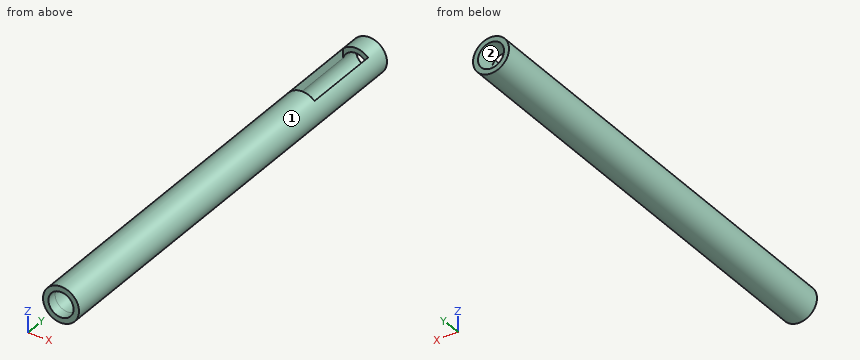
from build123d import *

# Parameters (mm, degrees)
SKETCH1_R           = 18
SKETCH1_R_2         = 13
BOSS_EXTRUDE1_DEPTH = 225
SKETCH8_R           = 18
BOSS_EXTRUDE3_DEPTH = 10
SKETCH9_R           = 12.55
CUT_EXTRUDE2_DEPTH  = 899.5
SKETCH23_W          = 25
SKETCH23_H          = 80
CUT_EXTRUDE16_DEPTH = 30


with BuildPart() as part:
    # Sketch1 → Boss-Extrude1 (new, symmetric)
    with BuildSketch(Plane(origin=(0, 0, 0), x_dir=(1, 0, 0), z_dir=(0, 1, 0))):
        with Locations(Location((0, 0, 0), (0, 0, 270))):
            Circle(SKETCH1_R)
        with Locations(Location((0, 0, 0), (0, 0, 270))):
            Circle(SKETCH1_R_2, mode=Mode.SUBTRACT)
    extrude(amount=BOSS_EXTRUDE1_DEPTH, both=True)

    # Sketch8 → Boss-Extrude3 (add)
    with BuildSketch(Plane.XZ.offset(225)):
        with Locations(Location((0, 0, 0), (0, 0, 270))):
            Circle(SKETCH8_R)
    extrude(amount=BOSS_EXTRUDE3_DEPTH)

    # Sketch9 → Cut-Extrude2 (cut)
    with BuildSketch(Plane(origin=(-32.302786122, 416.289190775, -45.221901395), x_dir=(-0.9768887275019512, 0, 0.2137484832217963), z_dir=(0, 1, 0))):
        with Locations(Location((-21.890114798, 51.081437247, 0), (0, 0, 257.657886074))):
            Circle(SKETCH9_R)
    extrude(amount=-CUT_EXTRUDE2_DEPTH, mode=Mode.SUBTRACT)

    # Sketch23 → Cut-Extrude16 (cut)
    with BuildSketch(Plane.XY):
        with Locations((0, 165)):
            Rectangle(SKETCH23_W, SKETCH23_H)
    extrude(amount=CUT_EXTRUDE16_DEPTH, mode=Mode.SUBTRACT)


solid = part.part
Design review of the part built by this model. Coordinates are the model's own, in mm. Face numbers are marked on the shaded views. Coordinates: 2 decimals unless noted, no trailing zeros. Write each loop counter-clockwise with the first axis right and the second up, starting at its lowest first coordinate (ties: lowest second). Pieces come first, ordered by that corner, then holes. Notation, with made-up numbers: (77, 39.25) - (85, 39.25) arc R9 ccw to (85, 56.25) - close; hole circle Ø1 at (51, -9.75). An arc over 180 degrees is marked (long way). One line per item, written item: value.
1) Add section C-C (y = 42). State the section outline as (x, z) points, plus the area to 3 significant figures.
Answer sheet:
outline: circle Ø36 at (0, 0); hole circle Ø26 at (0, 0)
area: 487 mm2
2) Mouldability with a two-part tool opening along X and no side actions: class the marked faces 1 and 2 as +X half, -X half, draft (parallel to the pull), parting line (faces both ways), or undercut.
Answer sheet:
face 1: parting line
face 2: undercut
3) Add section A-A (x = 0). State the section outline as (y, z) points.
Answer sheet:
outline: (-235, -18) - (225, -18) - (225, -13) - (-225, -13) - (-225, -12.55) - (-235, -12.55) - close; (-235, 12.55) - (-225, 12.55) - (-225, 13) - (125, 13) - (125, 18) - (-235, 18) - close; (205, 13) - (225, 13) - (225, 18) - (205, 18) - close
4) Insertion check: pin 1 (7.5 mm diameter, centred on y = 158.5, z = 9.5, fed in from -X); pin 2 (10.5 mm diameter, centred on y = 170, z = 7.5, fed in from +X); pin 3 (8 mm diameter, centred on x = 1.5, z = -6, fed in from +Y); pin 4 (1 mm diameter, centred on x = -10.5, y = -100, fed in from +Z). Each pin has a flat end and moves straight along its axis. Give the tip position at first contact, or say it passes through.
Answer sheet:
pin 1: stops at x = -17.06
pin 2: stops at x = 17.86
pin 3: passes through
pin 4: stops at z = 14.97
5) Add section B-B (z = -8.5). State the section outline as (x, y) points.
Answer sheet:
outline: (-15.87, -235) - (-9.23, -235) - (-9.23, -225) - (-9.84, -225) - (-9.84, 225) - (-15.87, 225) - close; (9.23, -235) - (15.87, -235) - (15.87, 225) - (9.84, 225) - (9.84, -225) - (9.23, -225) - close
6) To check wall thickness, follow probe 1 along X at (y, z) = (-2, 0); probe 2 along X at (y, z) = (-228.5, 0); probe 3 along Y at (x, z) = (7, 16.5). State the ranges of each line that lie inside material, in increasing order.
Answer sheet:
probe 1: x = -18 to -13, 13 to 18
probe 2: x = -18 to -12.55, 12.55 to 18
probe 3: y = -235 to 125, 205 to 225
